Part print with two shaded views. Sizes in mm from the minimum x, y, z corner. A direction names the side the tool comes from. Round coordinates to 2 decimals unless told otherwise and drop trailing zeros. Loops run counter-clockwise (first coordinate to the right, second up) from the corner with the lowest first, then second, coordinate; pieces in that order, holes last. Notation, with made-up numbers: M -1,89 L 11,89 A3 cw 11,93 Z; hole C 55,-11 d2. An arc over 180 degrees is marked long. Put each result on its own line as item: value. Start each with the question number.
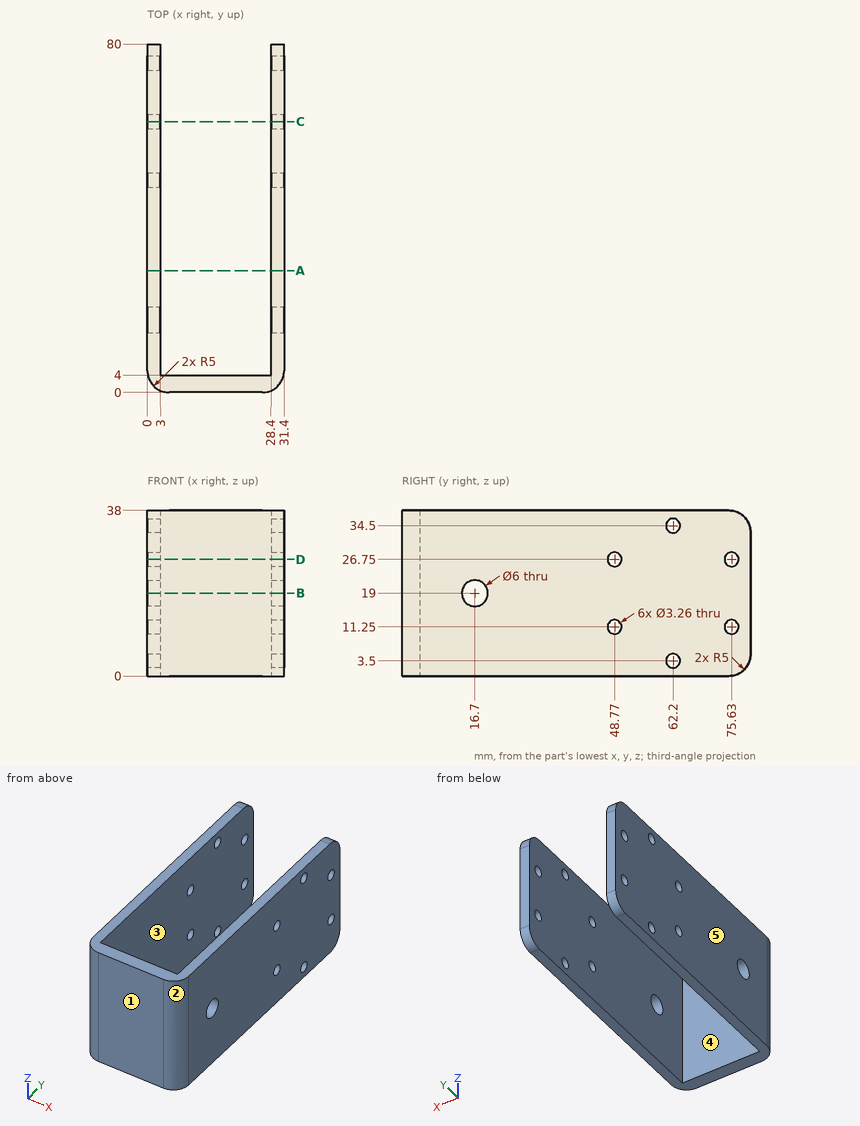
(1) Mould opens along X. For the marked faces 1, 2 and 3 say: +X half, -X half, draft (parallel to the pull), parting line (faces both ways), or undercut.
(2) Cut at B-B on z = 19. List the corners of the cut face in (x, y), and give its area (3 significant figures).
(3) Cut at D-D on z = 26.75. List the corners of the cut face in (x, y), and give its area (3 significant figures).
(4) Drill centre lines: line 1 along X through (y, z) = (18.5, 35.5); line 2 along Z through (x, y) = (29.5, 49.5); line 3 along Y through (x, z) = (29.8, 11.25). Where is each one in solid material? Low to high.
(5) Tool access for the marked faces 4 and 5: list every direction of +Z, -Z, +X, -X, +Y, -Y with a clear straight run to the whole face (end or side of a thin tool).
(6) Cut at C-C on y = 62.2. List the corners of the cut face in (x, z).
(7) Cut at A-A on y = 28. List the corners of the cut face in (x, z), and give its area (3 significant figures).
(8) Flat gauge pins, fed straight in: pin 1 Ø5 at (y, z) = (75.63, 11.25) entering from -X; pin 2 Ø12 at (x, y) = (10.5, 38) entering from +Z; pin 3 Ø1.5 at (x, z) = (7, 6.5) entering from +Y. Where does each tip first touch, or does it go through?
Taken from the geometry:
1. face 1: draft
1. face 2: +X half
1. face 3: undercut
2. outline: M 0,5 A5 ccw 5,0 L 26.4,0 A5 ccw 31.4,5 L 31.4,13.7 L 28.4,13.7 L 28.4,4 L 3,4 L 3,13.7 L 0,13.7 Z; M 0,19.7 L 3,19.7 L 3,80 L 0,80 Z; M 28.4,19.7 L 31.4,19.7 L 31.4,80 L 28.4,80 Z
2. area: 535 mm2
3. outline: M 0,5 A5 ccw 5,0 L 26.4,0 A5 ccw 31.4,5 L 31.4,47.14 L 28.4,47.14 L 28.4,4 L 3,4 L 3,47.14 L 0,47.14 Z; M 0,50.4 L 3,50.4 L 3,74 L 0,74 Z; M 0,77.26 L 3,77.26 L 3,80 L 0,80 Z; M 28.4,50.4 L 31.4,50.4 L 31.4,74 L 28.4,74 Z; M 28.4,77.26 L 31.4,77.26 L 31.4,80 L 28.4,80 Z
3. area: 532 mm2
4. line 1: 0 to 3, 28.4 to 31.4
4. line 2: 0 to 9.79, 12.71 to 25.29, 28.21 to 38
4. line 3: 1.33 to 47.14, 50.4 to 74, 77.26 to 80
5. face 4: +Z, -Z, +Y
5. face 5: +Z, -Z, -X, +Y, -Y
6. outline: M 0,0 L 3,0 L 3,1.87 L 0,1.87 Z; M 0,5.13 L 3,5.13 L 3,32.87 L 0,32.87 Z; M 0,36.13 L 3,36.13 L 3,38 L 0,38 Z; M 28.4,0 L 31.4,0 L 31.4,1.87 L 28.4,1.87 Z; M 28.4,5.13 L 31.4,5.13 L 31.4,32.87 L 28.4,32.87 Z; M 28.4,36.13 L 31.4,36.13 L 31.4,38 L 28.4,38 Z
7. outline: M 0,0 L 3,0 L 3,38 L 0,38 Z; M 28.4,0 L 31.4,0 L 31.4,38 L 28.4,38 Z
7. area: 228 mm2
8. pin 1: x = 0
8. pin 2: through
8. pin 3: y = 4
